Design review of the part built by this model. Coordinates are the model's own, in mm. A direction names the side the tool comes from. Round coordinates to 2 decimals unless told otherwise and drop trailing zeros. Loops run counter-clockwise (first coordinate to the right, second up) from the corner with the lowest first, then second, coordinate; pieces in that order, holes last. Notation, with made-up numbers: (19, 63.25) - (37, 63.25) arc R25 ccw to (37, 85.25) - close; hole circle Ø8 at (-37, 23.5). An arc over 180 degrees is marked (long way). One line per question, with ' | ' between items. Start each with the question number.
from build123d import *

# Parameters (mm, degrees)
BOSS_EXTRUDE1_START = 5
SKETCH2_R           = 30
SKETCH2_W           = 36
SKETCH2_H           = 36
SKETCH2_W_2         = 32
SKETCH2_H_2         = 32
BOSS_EXTRUDE1_DEPTH = 5
FILLET1_R           = 2
SKETCH3_2_R         = 1.75
CUT_EXTRUDE3_DEPTH  = 50.244289009
CUT_EXTRUDE4_DEPTH  = 1.5


with BuildPart() as part:
    # Sketch1 → Revolve1 (revolve)
    with BuildSketch(Plane(origin=(0, 0, 0), x_dir=(0, 0, -1), z_dir=(1, 0, 0)), mode=Mode.PRIVATE) as revolve1_sk:
        Polygon((-16, 30), (0, 30), (0, 7.15), (-8, 7.15), (-8, 9.15), (-10, 9.15), (-10, 11.15), (-12, 11.15), (-12, 13.15), (-14, 13.15), (-14, 15.15), (-16, 15.15), (-16, 17.15), (-18, 17.15), (-18, 19.15), (-20, 19.15), (-20, 21), (-16, 21), align=None)
    revolve(revolve1_sk.sketch.rotate(Axis((0, 0, 0), (0, 0, -1)), 90), axis=Axis((0, 0, 0), (0, 0, -1)))

    # Sketch2 → Boss-Extrude1 (add)
    # profile 1 of 2: a face of its own
    with BuildSketch(Plane(origin=(0, 0, 0), x_dir=(-1, 0, 0), z_dir=(0, 0, -1)).offset(BOSS_EXTRUDE1_START)):
        with Locations(Location((0, 0, 0), (0, 0, 180))):
            Circle(SKETCH2_R)
        Rectangle(SKETCH2_W, SKETCH2_H, mode=Mode.SUBTRACT)
    # profile 2 of 2: a face of its own
    with BuildSketch(Plane(origin=(0, 0, 0), x_dir=(-1, 0, 0), z_dir=(0, 0, -1)).offset(BOSS_EXTRUDE1_START)):
        Rectangle(SKETCH2_W, SKETCH2_H)
        Rectangle(SKETCH2_W_2, SKETCH2_H_2, mode=Mode.SUBTRACT)
    extrude(amount=-BOSS_EXTRUDE1_DEPTH)

    # Fillet1
    fillet1_edges = [part.edges().sort_by_distance(p)[0] for p in [
        (-16, 16, -2.5),
        (-16, -16, -2.5),
        (16, -16, -2.5),
        (16, 16, -2.5),
    ]]
    fillet(fillet1_edges, radius=FILLET1_R)

    # Sketch3_2 → Cut-Extrude3 (cut, through all)
    with BuildSketch(Plane(origin=(0, 0, -5), x_dir=(-1, 0, 0), z_dir=(0, 0, -1))):
        with Locations((-27, 0)):
            Circle(SKETCH3_2_R)
        with Locations((27, 0)):
            Circle(SKETCH3_2_R)
    extrude(amount=-CUT_EXTRUDE3_DEPTH, mode=Mode.SUBTRACT)

    # Sketch4 → Cut-Extrude4 (cut)
    with BuildSketch(Plane(origin=(0, 0, 0), x_dir=(-1, 0, 0), z_dir=(0, 0, -1))):
        with BuildLine():
            Line((-12.15, -8.65), (12.15, -8.65))
            ThreePointArc((12.15, -8.65), (13.564213562, -8.064213562), (14.15, -6.65))
            Line((14.15, -6.65), (14.15, 6.65))
            ThreePointArc((14.15, 6.65), (13.564213562, 8.064213562), (12.15, 8.65))
            Line((12.15, 8.65), (-12.15, 8.65))
            ThreePointArc((-12.15, 8.65), (-13.564213562, 8.064213562), (-14.15, 6.65))
            Line((-14.15, 6.65), (-14.15, -6.65))
            ThreePointArc((-14.15, -6.65), (-13.564213562, -8.064213562), (-12.15, -8.65))
        make_face()
    extrude(amount=-CUT_EXTRUDE4_DEPTH, mode=Mode.SUBTRACT)


solid = part.part
1. Take a section at C-C, the plane x = 27. Give the boundary of the cut face in (y, z).
2. Clearance check with flat-ended pins moving along their axes: P1, Ø6, axis at x = 22, z = 5, coming from the +Y side; P2, Ø11, axis at x = 3.5, y = 5.5, coming from the +Z side; P3, Ø1, axis at x = -14, z = 3, coming from the -Y side. State where each tip first meets the part, or that it passes through.
3. Take a section at B-B, the plane y = 0. Count the separate pieces of the cut face and the enclosed holes in it, then the cut area to 3 significant figures.
4. To check wall thickness, follow line 1 along Y through (x, z) = (-0.5, 17.5); line 2 along Y through (x, z) = (0, 13.35); line 3 along Z through (x, y) = (-12, -19). State the ranges of each line that lie inside material, in increasing order.
5. Take a section at A-A, the plane z = 4.5. Give the boundary of the cut face in (x, y), then the cut area to 3 significant figures.
6. Take a section at D-D, the plane y = 18. Give the boundary of the cut face in (x, z).
7. The part is to be moulded in two halves that separate along X. For faces 4 (the face through (14.15, 0, 1)), 5 (the face through (20.03, -6.31, 17.97)), 6 (the face through (5, 19, 20)), say which applies: pulls with the +X half, pulls with the -X half, needs draft (parallel to the pull), parting line crosses it, or undercut.
8. Machinability: for faces 1 (the face through (0, 8.65, 1)), 2 (the face through (-6.2, -20.4, 16)), 3 (the face through (28.75, 0.08, 5.35)), which of the approach directions +Z, -Z, +X, -X, +Y, -Y give a long, thin tool a straight path to every point of the face, cutting with its end or side? Answer none if there is none.
Answer list:
1) outline: (-13.08, -5) - (-1.75, -5) - (-1.75, 16) - (-13.08, 16) - close; (1.75, -5) - (13.08, -5) - (13.08, 16) - (1.75, 16) - close
2) P1: stops at y = 23.22 | P2: stops at z = 12 | P3: stops at y = -26.79
3) separate pieces: 4 | enclosed holes: 0 | area: 646 mm²
4) line 1: y = -20.99 to -17.14, 17.14 to 20.99 | line 2: y = -30 to -13.15, 13.15 to 30 | line 3: z = -5 to 16
5) outline: circle Ø60 at (0, 0); hole circle Ø3.5 at (-27, 0); hole circle Ø14.3 at (0, 0); hole circle Ø3.5 at (27, 0) | area: 2,650 mm²
6) outline: (-24, -5) - (24, -5) - (24, 16) - (10.82, 16) - (10.82, 20) - (6.54, 20) - (6.54, 18) - (-6.54, 18) - (-6.54, 20) - (-10.82, 20) - (-10.82, 16) - (-24, 16) - close
7) face 4: undercut | face 5: parting line crosses it | face 6: needs draft
8) face 1: -Z | face 2: +Z | face 3: +Z, -Z
